For this review, use the dimensioned drawing (mm, ordinates from the lowest corner) and the shaded views. A direction names the side the tool comes from. Coordinates: 2 decimals unless noted, no trailing zeros. Order: outer loops, then holes, each group sorted by start corner. A loop starts at its lowest first (then second) coordinate and runs counter-clockwise, first axis right, second up. Notation, with made-up numbers: M -10,50 L 24,50 A24 ccw 24,76 Z; hole C 70,89.5 d1. An arc over 180 degrees is marked long. Answer as CSV lines item,"result". Start each with the question number.
Q1. Consider section A-A on y = 5.1. Write out the cut boundary in (x, z).
Q2. Consider section D-D on y = 0.5. Write out the cut boundary in (x, z), and give its area (3 significant figures).
Q3. Machinability: for the marked faces 1, 2 and 3, which of the approach directions +Z, -Z, +X, -X, +Y, -Y give a long, thin tool a straight path to every point of the face, cutting with its end or side? Answer none if there is none.
Q4. Wall thickness on L1, parallel to Z at x = 19, y = 2.5; L2, parallel to Y at x = 38, z = 8; L3, parallel to Z at x = 2.9, y = 7.5: over which ranges is each line inside the solid? List them lowest first. Write a range as [from, to].
Q5. For P1, Ø2, axis at x = 38, y = 5.1, coming from the +Z side; P2, Ø1.1, axis at y = 4, z = 1.5, coming from the -X side; P3, Ø3, axis at x = 36, y = 4.5, coming from the -Z side; P4, Ø8, axis at x = 15, z = 7, coming from the -Y side, all flat-tipped, find the tip position at first contact; note any pin that passes through.
Q6. Consider section C-C on z = 16.15. Write out the cut boundary in (x, y).
Q7. Consider section B-B on x = 2.9. Write out the cut boundary in (y, z).
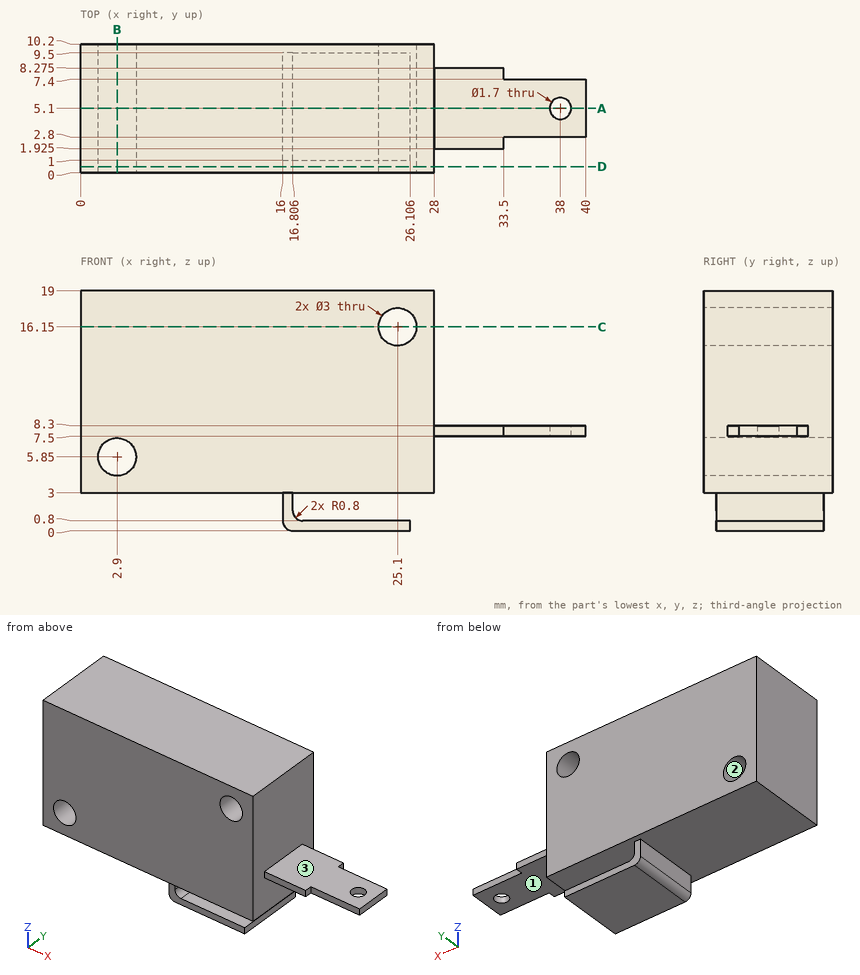
Evaluation:
1,outline,"M 0,3 L 16,3 L 16,0.8 A0.8 ccw 16.8,0 L 26.11,0 L 26.11,0.8 L 17.61,0.8 A0.8 cw 16.81,1.6 L 16.81,3 L 28,3 L 28,7.5 L 37.15,7.5 L 37.15,8.3 L 28,8.3 L 28,19 L 0,19 Z; M 38.85,7.5 L 40,7.5 L 40,8.3 L 38.85,8.3 Z; hole C 2.9,5.85 d3; hole C 25.1,16.15 d3"
2,outline,"M 0,3 L 28,3 L 28,19 L 0,19 Z; hole C 2.9,5.85 d3; hole C 25.1,16.15 d3"
2,area,"434 mm²"
3,face 1,"-Z, +X, +Y, -Y"
3,face 2,"+Y, -Y"
3,face 3,"+Z, +X, +Y, -Y"
4,L1,"z = [0, 0.8], [3, 19]"
4,L2,"y = [2.8, 4.25], [5.95, 7.4]"
4,L3,"z = [3, 4.35], [7.35, 19]"
5,P1,"stops at z = 8.3"
5,P2,"stops at x = 16"
5,P3,"stops at z = 7.5"
5,P4,"stops at y = 0"
6,outline,"M 0,0 L 23.6,0 L 23.6,10.2 L 0,10.2 Z; M 26.6,0 L 28,0 L 28,10.2 L 26.6,10.2 Z"
7,outline,"M 0,3 L 10.2,3 L 10.2,4.35 L 0,4.35 Z; M 0,7.35 L 10.2,7.35 L 10.2,19 L 0,19 Z"
